Can you work these out from the model? Positions are in its coordinate system, mm. Coordinates: 2 decimals unless noted, no trailing zeros. Loops run counter-clockwise (first coordinate to the right, second up) from the corner with the lowest first, then second, coordinate; pieces in that order, holes last.
Autodesk Inventor part; units mm, degrees
ref_plane "Work Plane1" through (19.05, 0, 0) normal (1, 0, 0) x (0, 0, -1)
ref_plane "YZ Plane" through (0, 0, 0) normal (1, 0, 0) x (0, 1, 0)
ref_plane "XZ Plane" through (0, 0, 0) normal (0, 1, 0) x (-1, 0, 0)
sketch "Sketch1" plane through (0, 0, 0) normal (0, 0, 1) x (1, 0, 0)
  line L0 (0, 0) -> (38.1, 0)
  line L1 (38.1, 0) -> (38.1, 50.8)
  line L2 (38.1, 50.8) -> (0, 50.8)
  line L3 (0, 50.8) -> (0, 0)
  dimension "d0" = 38.1
  dimension "d1" = 50.8
extrude "Extrusion1" add sketch "Sketch1" along normal blind 10.795
sketch "Sketch2" plane through (0, 0, 10.795) normal (0, 0, 1) x (1, 0, 0)
  line L0 (38.1, 0) -> (38.1, 50.8)
  line L1 (0, 0) -> (38.1, 0)
  circle A0 centre (35.052, 6.731) radius 1.4605
  circle A1 centre (35.052, 22.733) radius 1.4605
  dimension "d4" = 3.048
  dimension "d5" = 3.048
  dimension "d6" = 16.002
  dimension "d7" = 6.731
  dimension "d8" = 2.921
  dimension "d9" = 2.921
extrude "Extrusion2" cut sketch "Sketch2" against normal through all
ref_plane "Work Plane1" through (19.05, 0, 0) normal (1, 0, 0) x (0, 0, -1)
mirror "Mirror1" about plane through (19.05, 0, 0) normal (1, 0, 0) of "Extrusion2"
properties part number "Motor spacer"
Item 1: We'd pull the mould along Y, two halves only. Please class faces 1 (the face through (38.1, 25, 5)), 2 (the face through (19, 0, 5)), 3 (the face through (19, 50.8, 5)), 4 (the face through (1.7, 7.29, 5.47)): +Y half, -Y half, draft (parallel to the pull), parting line (faces both ways), or undercut.
Results are:
face 1: draft
face 2: -Y half
face 3: +Y half
face 4: undercut
Item 2: I'm going to push flat-ended pins straight in: P1, Ø4.5, axis at x = 35.052, y = 22.733, coming from the +Z side (3 decimals); P2, Ø2.5, axis at x = 3.048, y = 6.731, coming from the +Z side. Where does each tip first touch, or does it pass through?
Results are:
P1: stops at z = 10.795
P2: passes through
Item 3: Suppose I cut it at A-A, the plane x = 3. Please give me the cut outline in (y, z) (3 decimals).
Results are:
outline: (0, 0) - (5.271, 0) - (5.271, 10.795) - (0, 10.795) - close; (8.191, 0) - (21.273, 0) - (21.273, 10.795) - (8.191, 10.795) - close; (24.193, 0) - (50.8, 0) - (50.8, 10.795) - (24.193, 10.795) - close
Item 4: I need wall thicknesses on line 1 along Y through (x, z) = (34, 8.25); line 2 along Y through (x, z) = (3, 6.25); line 3 along X through (y, z) = (22, 2.5). Which ranges of each line are inside material? Lowest first, please.
Results are:
line 1: y = 0 to 5.72, 7.74 to 21.72, 23.75 to 50.8
line 2: y = 0 to 5.27, 8.19 to 21.27, 24.19 to 50.8
line 3: x = 0 to 1.78, 4.31 to 33.79, 36.32 to 38.1
